Part print with two shaded views. Sizes in mm from the minimum x, y, z corner. A direction names the side the tool comes from. Give positions to 0.01 mm unless a question says otherwise; leave off trailing zeros. Write each loop counter-clockwise with the first axis right and the second up, starting at its lowest first coordinate (ties: lowest second). Pieces come first, ordered by that corner, then holes.
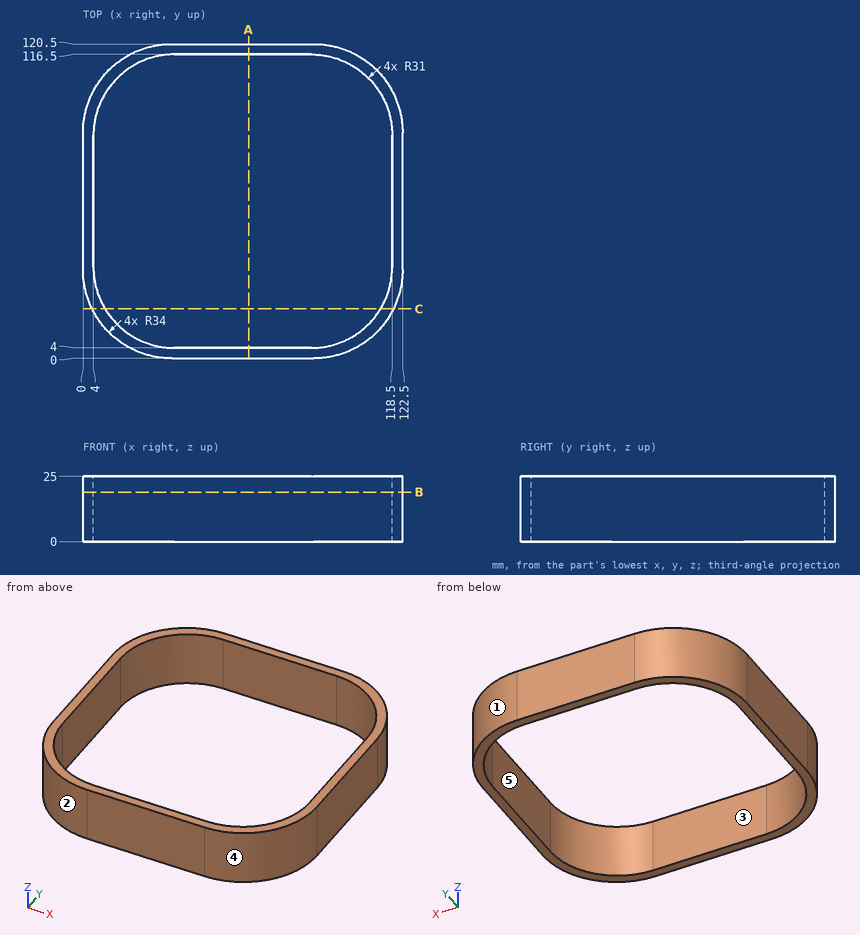
1) Drill centre lines: L1, parallel to X at y = 53.5, z = 17.75; L2, parallel to Y at x = 85, z = 3.25; L3, parallel to Y at x = 16.5, z = 10.25. Where is each one in solid material? Low to high.
Check result:
L1: x = 0 to 4, 118.5 to 122.5
L2: y = 0 to 4, 116.5 to 120.5
L3: y = 4.85 to 10.13, 110.37 to 115.65
2) Saw through at A-A (x = 63.5). Write the cut outline in (y, z), and give its area (3 significant figures).
Check result:
outline: (0, 0) - (4, 0) - (4, 25) - (0, 25) - close; (116.5, 0) - (120.5, 0) - (120.5, 25) - (116.5, 25) - close
area: 200 mm2
3) Mould opens along Y. For the marked faces 1, 2 and 3 say: +Y half, -Y half, draft (parallel to the pull), parting line (faces both ways), or undercut.
Check result:
face 1: +Y half
face 2: -Y half
face 3: undercut
4) Flat gauge pins, fed straight in: P1, Ø10, axis at y = 98.5, z = 7.5, coming from the -X side; P2, Ø5, axis at y = 105.5, z = 4.5, coming from the -X side. Where does each tip first touch, or does it go through?
Check result:
P1: stops at x = 0.73
P2: stops at x = 4.27
5) 3-axis set-ups, long thin cutter, end or side, ignore diameter. For the marked faces 4 and 5: which of +Z, -Z, +X, -X, +Y, -Y reach the whole face in a straight line?
Check result:
face 4: +Z, -Z, +X, -Y
face 5: +Z, -Z
6) Saw through at B-B (z = 19). Write the cut outline in (x, y), and give its area (3 significant figures).
Check result:
outline: (0, 34) arc R34 ccw to (34, 0) - (88.5, 0) arc R34 ccw to (122.5, 34) - (122.5, 86.5) arc R34 ccw to (88.5, 120.5) - (34, 120.5) arc R34 ccw to (0, 86.5) - close; hole (4, 35) arc R31 ccw to (35, 4) - (87.5, 4) arc R31 ccw to (118.5, 35) - (118.5, 85.5) arc R31 ccw to (87.5, 116.5) - (35, 116.5) arc R31 ccw to (4, 85.5) - close
area: 1,710 mm2
7) Saw through at C-C (y = 19). Write the cut outline in (x, z), and give its area (3 significant figures).
Check result:
outline: (3.49, 0) - (8.45, 0) - (8.45, 25) - (3.49, 25) - close; (114.05, 0) - (119.01, 0) - (119.01, 25) - (114.05, 25) - close
area: 248 mm2
